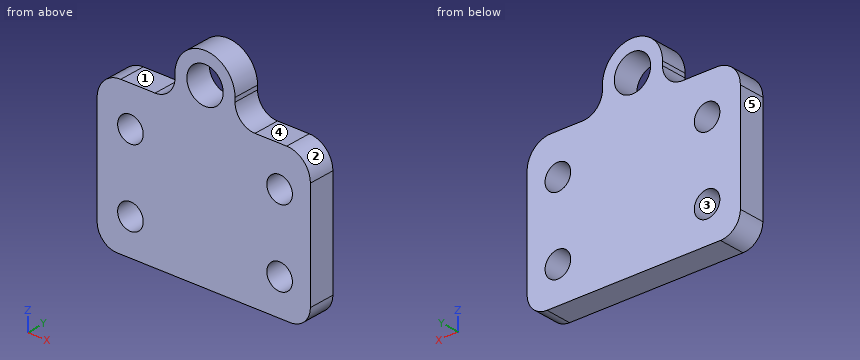
```python
from build123d import *

# Parameters (mm, degrees)
F0_R     = 3.212587
F0_R_2   = 4.561845
F1_DEPTH = 6.604


with BuildPart() as f1:
    # F0 (on Front) → F1 (new body)
    with BuildSketch(Plane.XZ):
        with BuildLine():
            Line((-48.562958, 0), (-5, 0))
            ThreePointArc((-5, 0), (-1.464466, 1.464466), (0, 5))
            Line((0, 5), (0, 31.923081))
            ThreePointArc((0, 31.923081), (-1.741241, 36.126808), (-5.944968, 37.868049))
            Line((-5.944968, 37.868049), (-13.91329, 37.868049))
            ThreePointArc((-13.91329, 37.868049), (-17.448823, 39.332515), (-18.91329, 42.868049))
            Line((-18.91329, 42.868049), (-18.91329, 43.906312))
            ThreePointArc((-18.91329, 43.906312), (-26.461123, 51.454146), (-34.008957, 43.906312))
            Line((-34.008957, 43.906312), (-34.008957, 42.868049))
            ThreePointArc((-34.008957, 42.868049), (-35.473424, 39.332515), (-39.008957, 37.868049))
            Line((-39.008957, 37.868049), (-47.61799, 37.868049))
            ThreePointArc((-47.61799, 37.868049), (-51.821717, 36.126808), (-53.562958, 31.923081))
            Line((-53.562958, 31.923081), (-53.562958, 5))
            ThreePointArc((-53.562958, 5), (-52.098492, 1.464466), (-48.562958, 0))
        make_face()
        with Locations((-45.20119, 9.01679)):
            Circle(F0_R, mode=Mode.SUBTRACT)
        with Locations((-7.721057, 9.01679)):
            Circle(F0_R, mode=Mode.SUBTRACT)
        with Locations((-45.20119, 27.906291)):
            Circle(F0_R, mode=Mode.SUBTRACT)
        with Locations((-7.721057, 27.906291)):
            Circle(F0_R, mode=Mode.SUBTRACT)
        with Locations((-26.461123, 43.906312)):
            Circle(F0_R_2, mode=Mode.SUBTRACT)
    extrude(amount=-F1_DEPTH)


solid = f1.part
```
Verification items for the finished model (mm, model axes). Face numbers are marked on the shaded views. A direction names the side the tool comes from. Round coordinates to 2 decimals unless told otherwise and drop trailing zeros. Write each loop counter-clockwise with the first axis right and the second up, starting at its lowest first coordinate (ties: lowest second). Pieces come first, ordered by that corner, then holes.
1. Section check D-D on z = 27. Enter the section's corners in (x, y), plus the area to 3 significant figures.
2. Access from +Z, -Z, +X, -X, +Y, -Y to the whole of each face (thin tool, end or side, straight path). Record for the marked faces 1 and 2.
3. Draft check along Z on the marked faces 3, 4 and 5. Enter one of: +Z half, -Z half, draft (parallel to the pull), parting line (faces both ways), or undercut.
4. Section check B-B on x = -23. Enter the section's corners in (y, z).
5. Section check A-A on z = 45. Enter the section's corners in (x, y), plus the area to 3 significant figures.
6. Section check C-C on y = 6. Enter the section's corners in (x, z).
7. Gauge pin test, flat ends, axial feed: P1, Ø3.5, axis at x = -11.5, y = 3, coming from the +Z side; P2, Ø6, axis at x = -7.72, z = 27.91, coming from the -Y side; P3, Ø0.5, axis at y = 3, z = 43.5, coming from the -X side; P4, Ø0.8, axis at y = 3.5, z = 43.5, coming from the +X side. Record the tip position at first contact, or that the pin passes through.
8. Scan lines: L1, parallel to Z at x = -45, y = 6.5; L2, parallel to X at y = 6.5, z = 8; L3, parallel to Z at x = -39, y = 5. Record each from-to range of solid material in increasing order.
Answer:
1. outline: (-53.56, 0) - (-48.28, 0) - (-48.28, 6.6) - (-53.56, 6.6) - close; (-42.12, 0) - (-10.8, 0) - (-10.8, 6.6) - (-42.12, 6.6) - close; (-4.64, 0) - (0, 0) - (0, 6.6) - (-4.64, 6.6) - close
1. area: 272 mm2
2. face 1: +Z, -X, +Y, -Y
2. face 2: +Z, +X, +Y, -Y
3. face 3: undercut
3. face 4: +Z half
3. face 5: draft
4. outline: (0, 0) - (6.6, 0) - (6.6, 40.93) - (0, 40.93) - close; (0, 46.88) - (6.6, 46.88) - (6.6, 50.61) - (0, 50.61) - close
5. outline: (-33.93, 0) - (-30.89, 0) - (-30.89, 6.6) - (-33.93, 6.6) - close; (-22.03, 0) - (-18.99, 0) - (-18.99, 6.6) - (-22.03, 6.6) - close
5. area: 40.1 mm2
6. outline: (-53.56, 5) arc R5 ccw to (-48.56, 0) - (-5, 0) arc R5 ccw to (0, 5) - (0, 31.92) arc R5.94 ccw to (-5.94, 37.87) - (-13.91, 37.87) arc R5 cw to (-18.91, 42.87) - (-18.91, 43.91) arc R7.55 ccw to (-34.01, 43.91) - (-34.01, 42.87) arc R5 cw to (-39.01, 37.87) - (-47.62, 37.87) arc R5.94 ccw to (-53.56, 31.92) - close; hole circle Ø6.43 at (-45.2, 9.02); hole circle Ø6.43 at (-45.2, 27.91); hole circle Ø9.12 at (-26.46, 43.91); hole circle Ø6.43 at (-7.72, 9.02); hole circle Ø6.43 at (-7.72, 27.91)
7. P1: stops at z = 37.87
7. P2: passes through
7. P3: stops at x = -34.01
7. P4: stops at x = -18.91
8. L1: z = 0 to 5.81, 12.22 to 24.7, 31.11 to 37.87
8. L2: x = -53.56 to -48.25, -42.15 to -10.77, -4.67 to 0
8. L3: z = 0 to 37.87
